Input: part model. Units: mm. Frame: model coordinates. Round coordinates to 2 decimals unless told otherwise and drop trailing zeros. Loops run counter-clockwise (first coordinate to the right, second up) from the corner with the lowest first, then second, coordinate; pieces in that order, holes last.
(1) First-contact query: pin 1 Ø2 at (x, z) = (-53.9, 12) entering from +Y. Flat tip, straight axial feed; report the tip coordinate or a pass-through.
(2) Cut plane B-B, the plane y = 1.35. Give the number of separate pieces and of enclosed holes in the cut face, and give its area (3 significant figures).
(3) Line query: line 1 (X direction, y = 0.8, z = -15); line 2 (X direction, y = 3.3, z = 12). Output: solid intervals per line, ascending.
(4) Cut plane C-C, the plane z = 15. Output: boundary loops of the cut face in (x, y), and give its area (3 significant figures).
(5) Cut plane A-A, the plane x = -15. Output: boundary loops of the cut face in (y, z).
from build123d import *

# Parameters (mm, degrees)
SKETCH1_W           = 127
SKETCH1_H           = 40
SKETCH1_R           = 1.2
SKETCH1_R_2         = 2.25
BOSS_EXTRUDE1_DEPTH = 6
SKETCH2_W           = 40
SKETCH2_H           = 6
CUT_EXTRUDE1_DEPTH  = 7
FILLET1_R           = 3


with BuildPart() as part:
    # Sketch1 → Boss-Extrude1 (new body)
    with BuildSketch(Plane(origin=(0, 0, 0), x_dir=(1, 0, 0), z_dir=(0, 1, 0))):
        Rectangle(SKETCH1_W, SKETCH1_H)
        with Locations(Location((60.5, 12, 0), (0, 0, 270))):
            Circle(SKETCH1_R, mode=Mode.SUBTRACT)
        with Locations(Location((-53.9, 12, 0), (0, 0, 270))):
            Circle(SKETCH1_R, mode=Mode.SUBTRACT)
        with Locations(Location((-15, 15, 0), (0, 0, 270))):
            Circle(SKETCH1_R_2, mode=Mode.SUBTRACT)
        with Locations(Location((15, 15, 0), (0, 0, 90))):
            Circle(SKETCH1_R_2, mode=Mode.SUBTRACT)
        with Locations(Location((60.5, -12, 0), (0, 0, 90))):
            Circle(SKETCH1_R, mode=Mode.SUBTRACT)
        with Locations(Location((15, -15, 0), (0, 0, 270))):
            Circle(SKETCH1_R_2, mode=Mode.SUBTRACT)
        with Locations(Location((-15, -15, 0), (0, 0, 90))):
            Circle(SKETCH1_R_2, mode=Mode.SUBTRACT)
        with Locations(Location((-53.9, -12, 0), (0, 0, 90))):
            Circle(SKETCH1_R, mode=Mode.SUBTRACT)
    extrude(amount=BOSS_EXTRUDE1_DEPTH)

    # Sketch2 → Cut-Extrude1 (cut)
    with BuildSketch(Plane.ZY.offset(63.5)):
        with Locations((0, 3)):
            Rectangle(SKETCH2_W, SKETCH2_H)
    extrude(amount=-CUT_EXTRUDE1_DEPTH, mode=Mode.SUBTRACT)

    # Fillet1
    fillet1_edges = [part.edges().sort_by_distance(p)[0] for p in [
        (-56.5, 3, -20),
        (-56.5, 3, 20),
        (63.5, 3, 20),
        (63.5, 3, -20),
    ]]
    fillet(fillet1_edges, radius=FILLET1_R)


solid = part.part
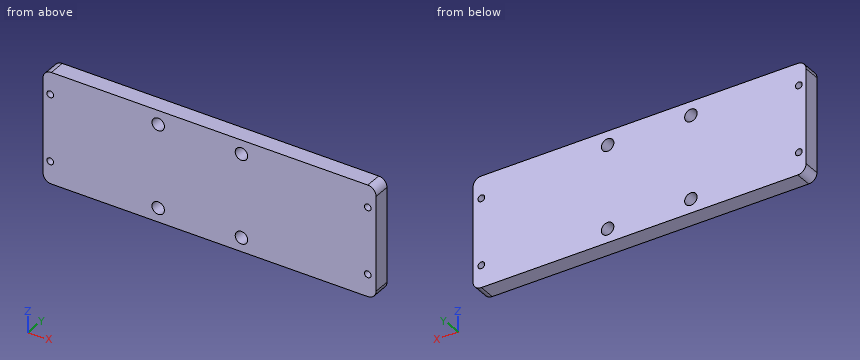
Reported:
1. pin 1: passes through
2. separate pieces: 1
2. enclosed holes: 8
2. area: 4,710 mm2
3. line 1: x = -56.5 to -17.25, -12.75 to 12.75, 17.25 to 63.5
3. line 2: x = -56.5 to -55.1, -52.7 to 59.3, 61.7 to 63.5
4. outline: (-56.5, 0) - (-17.25, 0) - (-17.25, 6) - (-56.5, 6) - close; (-12.75, 0) - (12.75, 0) - (12.75, 6) - (-12.75, 6) - close; (17.25, 0) - (63.5, 0) - (63.5, 6) - (17.25, 6) - close
4. area: 666 mm2
5. outline: (0, -20) - (6, -20) - (6, -17.25) - (0, -17.25) - close; (0, -12.75) - (6, -12.75) - (6, 12.75) - (0, 12.75) - close; (0, 17.25) - (6, 17.25) - (6, 20) - (0, 20) - close
